Drawing for the job (mm, zero at the part's lowest x, y, z). A direction names the side the tool comes from. Round coordinates to 2 decimals unless told otherwise and drop trailing zeros. Order: outer loops, then holes, each group sorted by start corner. A loop starts at its lowest first (then second) coordinate and runs counter-clockwise, first axis right, second up. Notation, with made-up numbers: (-27, 80.5) -> (24, 80.5) arc R13 cw to (24, 90.5) -> close; hole circle Ø4 at (18, -34.75). An arc over 180 degrees is marked (long way). Use CSV: the item, a comma, the result in double quotes.
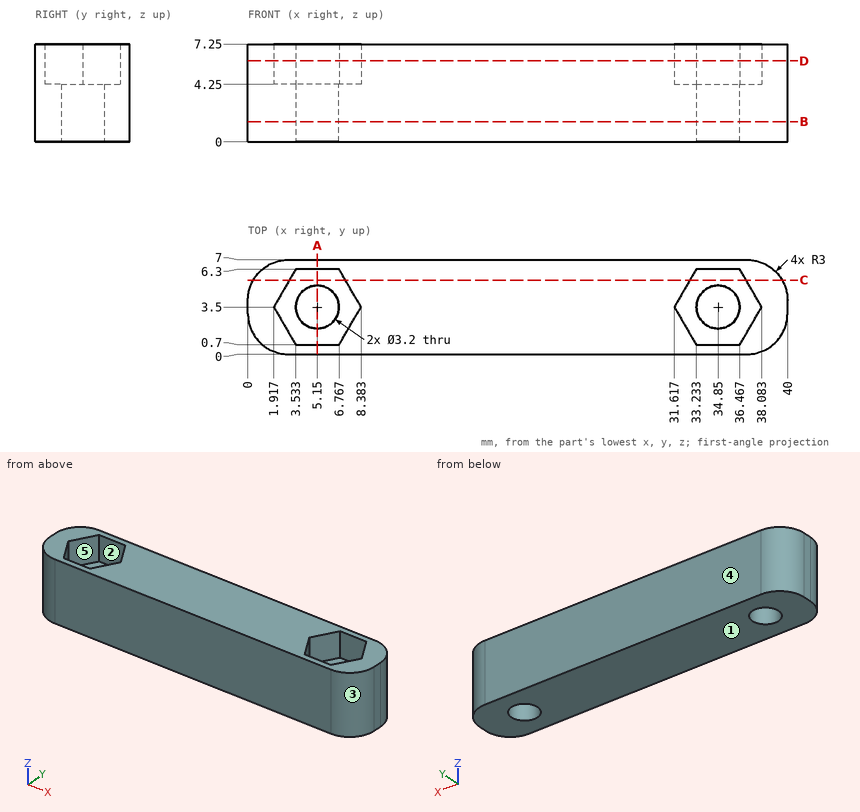
Q1. Mould opens along Y. For the marked faces 3, 4 and 5 say: +Y half, -Y half, draft (parallel to the pull), parting line (faces both ways), or undercut.
From the geometry:
face 3,"-Y half"
face 4,"+Y half"
face 5,"undercut"
Q2. Cut at B-B (z = 1.5). Give the cut face in (x, y), plus the area to 3 significant figures.
From the geometry:
outline,"(0, 3) arc R3 ccw to (3, 0) -> (37, 0) arc R3 ccw to (40, 3) -> (40, 4) arc R3 ccw to (37, 7) -> (3, 7) arc R3 ccw to (0, 4) -> close; hole circle Ø3.2 at (5.15, 3.5); hole circle Ø3.2 at (34.85, 3.5)"
area,"256 mm²"
Q3. Cut at C-C (y = 5.5). Give the cut face in (x, z).
From the geometry:
outline,"(0.4, 0) -> (39.6, 0) -> (39.6, 7.25) -> (36.93, 7.25) -> (36.93, 4.25) -> (32.77, 4.25) -> (32.77, 7.25) -> (7.23, 7.25) -> (7.23, 4.25) -> (3.07, 4.25) -> (3.07, 7.25) -> (0.4, 7.25) -> close"
Q4. Pin check, flat tips, straight feed: pin 1 (4 mm diameter, centred on x = 5.15, y = 3.5, fed in from +Z); pin 2 (3 mm diameter, centred on y = 2.5, z = 3, fed in from +X); pin 3 (3 mm diameter, centred on x = 34.85, y = 3.5, fed in from +Z); pin 4 (1.5 mm diameter, centred on y = 5, z = 6, fed in from -X). Stop position of each tip, or through.
From the geometry:
pin 1,"stops at z = 4.25"
pin 2,"stops at x = 40"
pin 3,"passes through"
pin 4,"stops at x = 0.01"
Q5. Probe line 1 along Y through (x, z) = (34.85, 3); line 2 along X through (y, z) = (2.5, 2.25); line 3 along X through (y, z) = (6, 5.5) (1 decimal). List the from-to ranges inside material, lowest first.
From the geometry:
line 1,"y = 0 to 1.9, 5.1 to 7"
line 2,"x = 0.04 to 3.9, 6.4 to 33.6, 36.1 to 39.96"
line 3,"x = 0.8 to 3.4, 6.9 to 33.1, 36.6 to 39.2"
Q6. Cut at D-D (z = 6). Give the cut face in (x, y), plus the area to 3 significant figures.
From the geometry:
outline,"(0, 3) arc R3 ccw to (3, 0) -> (37, 0) arc R3 ccw to (40, 3) -> (40, 4) arc R3 ccw to (37, 7) -> (3, 7) arc R3 ccw to (0, 4) -> close; hole (1.92, 3.5) -> (3.53, 0.7) -> (6.77, 0.7) -> (8.38, 3.5) -> (6.77, 6.3) -> (3.53, 6.3) -> close; hole (31.62, 3.5) -> (33.23, 0.7) -> (36.47, 0.7) -> (38.08, 3.5) -> (36.47, 6.3) -> (33.23, 6.3) -> close"
area,"218 mm²"
Q7. Cut at A-A (x = 5.15). Give the cut face in (y, z).
From the geometry:
outline,"(0, 0) -> (1.9, 0) -> (1.9, 4.25) -> (0.7, 4.25) -> (0.7, 7.25) -> (0, 7.25) -> close; (5.1, 0) -> (7, 0) -> (7, 7.25) -> (6.3, 7.25) -> (6.3, 4.25) -> (5.1, 4.25) -> close"
Q8. Which spindle directions (+Z, -Z, +X, -X, +Y, -Y) get a long thin tool onto all of the face, cutting with end or side? Do the marked faces 1 and 2. Say none if no direction does.
From the geometry:
face 1,"-Z, +X, -X, +Y, -Y"
face 2,"+Z"
